Can you work these out from the model? Positions are in its coordinate system, mm. A direction names the side the tool comes from. Coordinates: 2 decimals unless noted, no trailing zeros.
Autodesk Inventor part; units mm, degrees
ref_plane "YZ Plane" through (0, 0, 0) normal (1, 0, 0) x (0, 1, 0)
ref_plane "XZ Plane" through (0, 0, 0) normal (0, 1, 0) x (-1, 0, 0)
ref_plane "XY Plane" through (0, 0, 0) normal (0, 0, 1) x (1, 0, 0)
sketch "Sketch1" plane through (0, 0, 0) normal (0, 1, 0) x (-1, 0, 0)
  line L0 (0, 0) -> (30, 0)
  line L1 (30, 0) -> (30, -40)
  line L2 (30, -40) -> (0, -40)
  line L3 (0, -40) -> (0, 0)
  dimension "d0" = 30
  dimension "d1" = 40
extrude "Extrusion1" add sketch "Sketch1" along normal blind 30
sketch "Sketch6" plane through (0, 30, 0) normal (0, 1, 0) x (1, 0, 0)
  line L0 (0, 0) -> (-15, 0)
  line L1 (-30, 0) -> (0, 0)
  circle A0 centre (-15, 0) radius 1.5
  dimension "d32" = 3
extrude "Extrusion6" cut sketch "Sketch6" against normal blind 30
pattern_circular "Circular Pattern4" count 3 over 360 about axis through (-15, 30, 0) along (0, -1, 0) of "Extrusion1", "Extrusion6"
sketch "Sketch7" plane through (0, 0, -40) normal (0, 0, -1) x (-1, 0, 0)
  line L0 (4.5, 4.5) -> (25.5, 4.5)
  line L1 (25.5, 4.5) -> (25.5, 25.5)
  line L2 (25.5, 25.5) -> (4.5, 25.5)
  line L3 (4.5, 25.5) -> (4.5, 4.5)
  line L4 (15, 30) -> (15, 0)
  line L5 (4.5, 4.5) -> (25.5, 25.5) construction
  line L6 (25.5, 4.5) -> (4.5, 25.5) construction
  point P0 (0, 0)
  point P1 (15, 15)
  dimension "d38" = 21
  dimension "d39" = 21
extrude "Extrusion7" cut sketch "Sketch7" against normal blind 15
pattern_circular "Circular Pattern5" count 3 over 360 about axis through (-15, 30, 0) along (0, -1, 0) of "Extrusion7"
sketch "Sketch8" plane through (-15, 0, 17.3205) normal (-0.5, 0, 0.866) x (0.866, 0, 0.5)
  line L0 (31.3397, 0) -> (31.3397, 30)
  line L1 (31.3397, 15) -> (21.3397, 15)
  circle A0 centre (21.3397, 15) radius 2.75
  point P0 (4.3301, 0)
  dimension "d45" = 10
  dimension "d46" = 5.5
extrude "Extrusion8" cut sketch "Sketch8" against normal blind 30
pattern_circular "Circular Pattern6" count 3 over 360 about axis through (-15, 30, 0) along (0, -1, 0) of "Extrusion8"
fillet "Fillet5" radius 5 3 edges at (-15, 15, 17.3205) (0, 15, -8.6603) (-30, 15, -8.6603)
fillet "Fillet6" radius 5 6 edges at (-30, 30, -25.7735) (-44.8205, 30, -0.1036) (-0.1795, 30, 25.8771) (-29.8205, 30, 25.8771) (14.8205, 30, -0.1036) (0, 30, -25.7735)
fillet "Fillet7" radius 4 15 edges at (-28.5355, 28.5355, -40) (-30, 12.5, -40) (-1.4645, 28.5355, -40) (0, 12.5, -40) (-15, 30, -40) (-42.8732, 28.5355, 31.7221) (-42.141, 12.5, 32.9904) (-56.4088, 28.5355, 8.2779) (-57.141, 12.5, 7.0096) (-49.641, 30, 20) (26.4088, 28.5355, 8.2779) (27.141, 12.5, 7.0096) (12.8732, 28.5355, 31.7221) (12.141, 12.5, 32.9904) (19.641, 30, 20)
properties part number "80_20_top_connector"
(1) If we mould it in two halves opening along Y, with no side actions, what happens to faces 4 (the flat face through (-15, 15, -25)), 5 (the flat face through (-50.02, 4.27, 19.34)), 6 (the cylindrical face through (-1.347, 28.496, 23.557))? For each: released by +Y, released by -Y, zero draft, split by the parting line, or undercut.
Check values:
face 4: undercut
face 5: zero draft
face 6: released by +Y
(2) Which directions (+Z, -Z, +X, -X, +Y, -Y) give clear straight access to the entire face, cutting with the end or side of a thin tool? Please do faces 1 (the flat face through (-49.93, 15.147, 8.043)), 2 (the flat face through (-39.43, 14.85, 26.23)), 3 (the flat face through (-30, 12, -24)).
Check values:
face 1: none
face 2: -X
face 3: -Z, -X, +Y, -Y
(3) I'm going to push flat-ended pins straight in: pin 1 (3 mm diameter, centred on x = -9.5, y = 25, fed in from +Z); pin 2 (4.5 mm diameter, centred on y = 11.5, z = -31, fed in from -X); pin 3 (12 mm diameter, centred on x = -17.5, y = 17, fed in from +Z). Where does each tip first touch, or does it pass through?
Check values:
pin 1: stops at z = 21.36
pin 2: stops at x = -30
pin 3: stops at z = 22.23
(4) If I drill on probe 1 along Y at (x, z) = (6, 23); probe 2 along Z at (x, y) = (-15, 12.75); probe 3 along X at (y, z) = (13.5, 5.5), over which ranges is the centre line in solid material (lowest first)?
Check values:
probe 1: y = 0 to 4.5, 25.5 to 30
probe 2: z = -25 to -1.5, 1.5 to 18.09
probe 3: x = -54.35 to -49.13, -40.69 to 10.69, 19.13 to 24.35
(5) I want a section at B-B on y = 15. State how many separate pieces and enclosed holes the cut face has, then the cut area to 3 significant figures.
Check values:
separate pieces: 7
enclosed holes: 1
area: 2,090 mm2
